from build123d import *

# Parameters (mm, degrees)
ESQUISSE1_R             = 37
ESQUISSE1_R_2           = 2
ESQUISSE1_W             = 25
ESQUISSE1_H             = 3
BOSS_EXTRU_1_DEPTH      = 2
BOSS_EXTRU_2_DEPTH      = 15
ESQUISSE3_W             = 2
ESQUISSE3_H             = 28.4
BOSS_EXTRU_3_DEPTH      = 2.25
ESQUISSE5_W             = 2
ESQUISSE5_H             = 24.4
BOSS_EXTRU_4_DEPTH      = 2.25
ESQUISSE7_W             = 33.1
ESQUISSE7_H             = 28.4
BOSS_EXTRU_5_DEPTH      = 1
ESQUISSE8_W             = 15
ESQUISSE8_H             = 15
ENL_V_MAT_EXTRU_1_DEPTH = 3
ESQUISSE9_W             = 21
ESQUISSE9_H             = 2.5
ENL_V_MAT_EXTRU_2_DEPTH = 3
ESQUISSE11_W            = 33.1
ESQUISSE11_H            = 28.4
ENL_V_MAT_EXTRU_4_DEPTH = 15
SKETCH1_R               = 1.75
SKETCH1_R_2             = 1
BOSS_EXTRUDE1_DEPTH     = 10
CUT_EXTRUDE1_START      = -10
SKETCH1_3_R             = 1
CUT_EXTRUDE1_DEPTH      = 10


with BuildPart() as part:
    # Esquisse1 → Boss.-Extru.1 (new body)
    with BuildSketch(Plane.XY):
        Circle(ESQUISSE1_R)
        with Locations((0, 30)):
            Circle(ESQUISSE1_R_2, mode=Mode.SUBTRACT)
        with Locations((-22.874807889, 14.34375)):
            Circle(ESQUISSE1_R_2, mode=Mode.SUBTRACT)
        with Locations((-25.416453209, -15.9375)):
            Circle(ESQUISSE1_R_2, mode=Mode.SUBTRACT)
        with Locations((0, -27)):
            Circle(ESQUISSE1_R_2, mode=Mode.SUBTRACT)
        with Locations((25.416453209, -15.9375)):
            Circle(ESQUISSE1_R_2, mode=Mode.SUBTRACT)
        with Locations((22.874807889, 14.34375)):
            Circle(ESQUISSE1_R_2, mode=Mode.SUBTRACT)
        with Locations((0, -15.5)):
            Rectangle(ESQUISSE1_W, ESQUISSE1_H, mode=Mode.SUBTRACT)
    extrude(amount=BOSS_EXTRU_1_DEPTH)

    # Esquisse2 → Boss.-Extru.2 (add)
    with BuildSketch(Plane(origin=(0, 0, 0), x_dir=(-1, 0, 0), z_dir=(0, 0, -1))):
        Polygon((-16.55, 14.9), (-12.55, 14.9), (-12.55, -9.5), (12.55, -9.5), (12.55, 14.9), (16.55, 14.9), (16.55, -13.5), (-16.55, -13.5), align=None)
    extrude(amount=BOSS_EXTRU_2_DEPTH)

    # Esquisse3 → Boss.-Extru.3 (add)
    with BuildSketch(Plane(origin=(-12.55, 0, 0), x_dir=(0, 0, -1), z_dir=(1, 0, 0))):
        with Locations((9.625, 0.7)):
            Rectangle(ESQUISSE3_W, ESQUISSE3_H)
        with Locations((6.625, 0.7)):
            Rectangle(ESQUISSE3_W, ESQUISSE3_H)
    extrude(amount=BOSS_EXTRU_3_DEPTH)

    # Esquisse5 → Boss.-Extru.4 (add)
    with BuildSketch(Plane.ZY.offset(-12.55)):
        with Locations((-9.625, 2.7)):
            Rectangle(ESQUISSE5_W, ESQUISSE5_H)
        with Locations((-6.625, 2.7)):
            Rectangle(ESQUISSE5_W, ESQUISSE5_H)
    extrude(amount=BOSS_EXTRU_4_DEPTH)

    # Esquisse7 → Boss.-Extru.5 (add)
    with BuildSketch(Plane(origin=(0, 0, -15), x_dir=(-1, 0, 0), z_dir=(0, 0, -1))):
        with Locations((0, 0.7)):
            Rectangle(ESQUISSE7_W, ESQUISSE7_H)
    extrude(amount=-BOSS_EXTRU_5_DEPTH)

    # Esquisse8 → Enl_v. mat.-Extru.1 (cut)
    with BuildSketch(Plane(origin=(0, 0, -15), x_dir=(-1, 0, 0), z_dir=(0, 0, -1))):
        Rectangle(ESQUISSE8_W, ESQUISSE8_H)
    extrude(amount=-ENL_V_MAT_EXTRU_1_DEPTH, mode=Mode.SUBTRACT)

    # Esquisse9 → Enl_v. mat.-Extru.2 (cut)
    with BuildSketch(Plane.XZ.offset(13.5)):
        with Locations((0, -5.65)):
            Rectangle(ESQUISSE9_W, ESQUISSE9_H)
    extrude(amount=-ENL_V_MAT_EXTRU_2_DEPTH, mode=Mode.SUBTRACT)

    # Esquisse11 → Enl_v. mat.-Extru.4 (cut)
    with BuildSketch(Plane(origin=(0, 0, -15), x_dir=(-1, 0, 0), z_dir=(0, 0, -1))):
        with Locations((0, 0.7)):
            Rectangle(ESQUISSE11_W, ESQUISSE11_H)
    extrude(amount=-ENL_V_MAT_EXTRU_4_DEPTH, mode=Mode.SUBTRACT)

    # Sketch1 → Boss-Extrude1 (add)
    # profile 1 of 4: a face of its own
    with BuildSketch(Plane(origin=(0, 0, 0), x_dir=(-1, 0, 0), z_dir=(0, 0, -1))):
        with Locations(Location((7.9, -1.5, 0), (0, 0, 180))):
            Circle(SKETCH1_R)
        with Locations((7.9, -1.5)):
            Circle(SKETCH1_R_2, mode=Mode.SUBTRACT)
    # profile 2 of 4: a face of its own
    with BuildSketch(Plane(origin=(0, 0, 0), x_dir=(-1, 0, 0), z_dir=(0, 0, -1))):
        with Locations(Location((7.9, 11, 0), (0, 0, 180))):
            Circle(SKETCH1_R)
        with Locations((7.9, 11)):
            Circle(SKETCH1_R_2, mode=Mode.SUBTRACT)
    # profile 3 of 4: a face of its own
    with BuildSketch(Plane(origin=(0, 0, 0), x_dir=(-1, 0, 0), z_dir=(0, 0, -1))):
        with Locations(Location((-13.1, 11, 0), (0, 0, 180))):
            Circle(SKETCH1_R)
        with Locations((-13.1, 11)):
            Circle(SKETCH1_R_2, mode=Mode.SUBTRACT)
    # profile 4 of 4: a face of its own
    with BuildSketch(Plane(origin=(0, 0, 0), x_dir=(-1, 0, 0), z_dir=(0, 0, -1))):
        with Locations(Location((-13.1, -1.5, 0), (0, 0, 180))):
            Circle(SKETCH1_R)
        with Locations((-13.1, -1.5)):
            Circle(SKETCH1_R_2, mode=Mode.SUBTRACT)
    extrude(amount=BOSS_EXTRUDE1_DEPTH)

    # Sketch1_3 → Cut-Extrude1 (cut)
    with BuildSketch(Plane(origin=(0, 0, 0), x_dir=(-1, 0, 0), z_dir=(0, 0, -1)).offset(CUT_EXTRUDE1_START)):
        with Locations(Location((-13.1, 11, 0), (0, 0, 180))):
            Circle(SKETCH1_3_R)
        with Locations(Location((-13.1, -1.5, 0), (0, 0, 180))):
            Circle(SKETCH1_3_R)
        with Locations(Location((7.9, -1.5, 0), (0, 0, 180))):
            Circle(SKETCH1_3_R)
        with Locations(Location((7.9, 11, 0), (0, 0, 180))):
            Circle(SKETCH1_3_R)
    extrude(amount=CUT_EXTRUDE1_DEPTH, mode=Mode.SUBTRACT)


solid = part.part
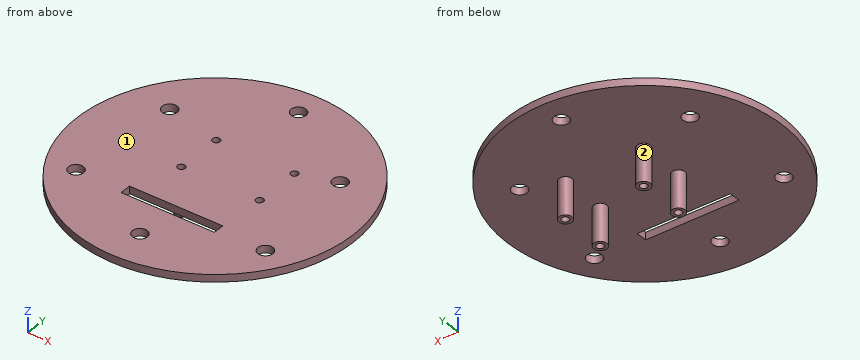
Check sheet for the modelled part. Datum: model origin and axes. Units: mm. Face numbers are marked on the shaded views. Coordinates: 2 decimals unless noted, no trailing zeros. Loops run counter-clockwise (first coordinate to the right, second up) from the corner with the lowest first, then second, coordinate; pieces in that order, holes last. Notation, with made-up numbers: (-10, 48) -> (30, 48) arc R16 cw to (30, 77) -> close; hole circle Ø9 at (-5, 84). An arc over 180 degrees is marked (long way). Answer in a Markdown table with one row per item.
1. Go/stop test with flat-tipped pins: pin 1 (1.6 mm diameter, centred on x = 13.1, y = -1.5, fed in from -Z); pin 2 (0.6 mm diameter, centred on y = -16, z = 0.5, fed in from +X); pin 3 (1.5 mm diameter, centred on x = 28, y = -22, fed in from -Z); pin 4 (4 mm diameter, centred on y = -2, z = -1, fed in from +X). Record where each tip stops, or that it passes through.
Check values:
| item | result |
|---|---|
| pin 1 | passes through |
| pin 2 | stops at x = 33.5 |
| pin 3 | stops at z = 0 |
| pin 4 | stops at x = 37 |
2. Sectioned sample at A-A, the plane z = -8.5. Record the boundary of the cut face in (x, y).
Check values:
| item | result |
|---|---|
| outline | circle Ø3.5 at (-7.9, -1.5); circle Ø3.5 at (-7.9, 11); circle Ø3.5 at (13.1, -1.5); circle Ø3.5 at (13.1, 11); hole circle Ø2 at (-7.9, -1.5); hole circle Ø2 at (-7.9, 11); hole circle Ø2 at (13.1, -1.5); hole circle Ø2 at (13.1, 11) |
3. Release check for a two-part mould opening along X. For the marked faces 1 and 2 record: released by +X, released by -X, zero draft, split by the parting line, or undercut.
Check values:
| item | result |
|---|---|
| face 1 | zero draft |
| face 2 | undercut |
4. Sectioned sample at C-C, the plane y = 30. Record the boundary of the cut face in (x, z), then the cut area to 3 significant figures.
Check values:
| item | result |
|---|---|
| outline | (-21.66, 0) -> (-2, 0) -> (-2, 2) -> (-21.66, 2) -> close; (2, 0) -> (21.66, 0) -> (21.66, 2) -> (2, 2) -> close |
| area | 78.6 mm2 |
5. Sectioned sample at D-D, the plane y = 11. Record the boundary of the cut face in (x, z).
Check values:
| item | result |
|---|---|
| outline | (-35.33, 0) -> (-9.65, 0) -> (-9.65, -10) -> (-8.9, -10) -> (-8.9, 2) -> (-35.33, 2) -> close; (-6.9, -10) -> (-6.15, -10) -> (-6.15, 0) -> (11.35, 0) -> (11.35, -10) -> (12.1, -10) -> (12.1, 2) -> (-6.9, 2) -> close; (14.1, -10) -> (14.85, -10) -> (14.85, 0) -> (35.33, 0) -> (35.33, 2) -> (14.1, 2) -> close |
6. Sectioned sample at B-B, the plane x = 0. Record the boundary of the cut face in (y, z).
Check values:
| item | result |
|---|---|
| outline | (-37, 0) -> (-29, 0) -> (-29, 2) -> (-37, 2) -> close; (-25, 0) -> (-17, 0) -> (-17, 2) -> (-25, 2) -> close; (-14, 0) -> (28, 0) -> (28, 2) -> (-14, 2) -> close; (32, 0) -> (37, 0) -> (37, 2) -> (32, 2) -> close |
7. Material ranges on line 1 along Y through (x, z) = (0, 1.5); line 2 along Y through (x, z) = (-8, -9.5); line 3 along Z through (x, y) = (-12, -21), recorded low to high. Write a range as [from, to].
Check values:
| item | result |
|---|---|
| line 1 | y = [-37, -29], [-25, -17], [-14, 28], [32, 37] |
| line 2 | y = [-3.25, -2.49], [-0.51, 0.25], [9.25, 10.01], [11.99, 12.75] |
| line 3 | z = [0, 2] |
